Part model, mm, in its own coordinate system. A direction names the side the tool comes from. Round coordinates to 2 decimals unless told otherwise and drop trailing zeros. Loops run counter-clockwise (first coordinate to the right, second up) from the corner with the lowest first, then second, coordinate; pieces in that order, holes last.
from build123d import *
from OCP.BRepFilletAPI import BRepFilletAPI_MakeChamfer

# Parameters (mm, degrees)
SKETCH1_W           = 82
SKETCH1_H           = 30
BOSS_EXTRUDE1_DEPTH = 5
CUT_EXTRUDE1_DEPTH  = 10
CHAMFER1_SIZE       = 0.5
CHAMFER1_SIZE2      = 0.366025404
CUT_EXTRUDE3_REACH  = 89.459
CHAMFER3_SIZE       = 0.5


with BuildPart() as part:
    # Sketch1 → Boss-Extrude1 (new body)
    with BuildSketch(Plane.XY):
        with Locations((41, 15)):
            Rectangle(SKETCH1_W, SKETCH1_H)
    extrude(amount=BOSS_EXTRUDE1_DEPTH)

    # Sketch2 → Cut-Extrude1 (cut)
    with BuildSketch(Plane.XZ):
        Polygon((0.973292227, 5.1), (9.093205081, 5.1), (6.090983681, -0.1), (3.975513627, -0.1), align=None)
        Polygon((9.860043573, -0.1), (17.979956427, -0.1), (14.977735027, 5.1), (12.862264973, 5.1), align=None)
        Polygon((18.743292227, 5.1), (26.863205081, 5.1), (23.860983681, -0.1), (21.745513627, -0.1), align=None)
        Polygon((27.630043573, -0.1), (35.749956427, -0.1), (32.747735027, 5.1), (30.632264973, 5.1), align=None)
        Polygon((36.513292227, 5.1), (44.633205081, 5.1), (41.630983681, -0.1), (39.515513627, -0.1), align=None)
        Polygon((45.400043573, -0.1), (53.519956427, -0.1), (50.517735027, 5.1), (48.402264973, 5.1), align=None)
        Polygon((54.283292227, 5.1), (62.403205081, 5.1), (59.400983681, -0.1), (57.285513627, -0.1), align=None)
        Polygon((63.170043573, -0.1), (71.289956427, -0.1), (68.287735027, 5.1), (66.172264973, 5.1), align=None)
        Polygon((72.053292227, 5.1), (80.173205081, 5.1), (77.170983681, -0.1), (75.055513627, -0.1), align=None)
    extrude(amount=-CUT_EXTRUDE1_DEPTH, mode=Mode.SUBTRACT)

    # Chamfer1: one chamfer whose edges measure the first distance from different faces: ONE call of the kernel's chamfer builder (chamfer() names one face for all edges)
    chamfer1_edges_1 = [part.edges().sort_by_distance(p)[0] for p in [
        (31.69, 10, 5),
        (40.573248654, 10, 5),
        (49.46, 10, 5),
        (58.343248654, 10, 5),
        (8.033248654, 0, 0),
        (67.23, 10, 5),
        (19.805, 0, 0),
        (25.803248654, 0, 0),
        (37.575, 0, 0),
        (76.113248654, 10, 5),
        (43.573248654, 0, 0),
        (55.345, 0, 0),
        (61.343248654, 0, 0),
        (73.115, 0, 0),
        (79.614359354, 0, 0),
        (76.113248654, 10, 0),
        (67.23, 10, 0),
        (58.343248654, 10, 0),
        (49.46, 10, 0),
        (40.573248654, 10, 0),
        (31.69, 10, 0),
        (22.803248654, 10, 0),
        (13.92, 10, 0),
        (5.033248654, 10, 0),
        (10.92, 0, 5),
        (16.918248654, 0, 5),
        (28.69, 0, 5),
        (34.688248654, 0, 5),
        (46.46, 0, 5),
        (52.458248654, 0, 5),
        (64.23, 0, 5),
        (70.228248654, 0, 5),
        (81.057735027, 0, 5),
        (1.9588893, 0, 0),
        (5.033248654, 10, 5),
        (13.92, 10, 5),
        (0.515513627, 0, 5),
        (22.803248654, 10, 5),
    ]]
    chamfer1_edges_2 = [part.edges().sort_by_distance(p)[0] for p in [
        (48.344529946, 5, 5),
    ]]
    chamfer1_side_2 = [part.faces().sort_by_distance(p)[0] for p in [
        (46.901154273, 5, 2.5),
    ]]
    chamfer1_edges_3 = [part.edges().sort_by_distance(p)[0] for p in [
        (50.575470054, 5, 5),
    ]]
    chamfer1_side_3 = [part.faces().sort_by_distance(p)[0] for p in [
        (52.018845727, 5, 2.5),
    ]]
    chamfer1_edges_4 = [part.edges().sort_by_distance(p)[0] for p in [
        (66.114529946, 5, 5),
    ]]
    chamfer1_side_4 = [part.faces().sort_by_distance(p)[0] for p in [
        (64.671154273, 5, 2.5),
    ]]
    chamfer1_edges_5 = [part.edges().sort_by_distance(p)[0] for p in [
        (68.345470054, 5, 5),
    ]]
    chamfer1_side_5 = [part.faces().sort_by_distance(p)[0] for p in [
        (69.788845727, 5, 2.5),
    ]]
    chamfer1_edges_6 = [part.edges().sort_by_distance(p)[0] for p in [
        (77.228718708, 5, 0),
        (74.9977786, 5, 0),
        (59.458718708, 5, 0),
        (57.2277786, 5, 0),
        (41.688718708, 5, 0),
        (39.4577786, 5, 0),
        (23.918718708, 5, 0),
        (21.6877786, 5, 0),
        (6.148718708, 5, 0),
        (3.9177786, 5, 0),
    ]]
    chamfer1_side_6 = [part.faces().sort_by_distance(p)[0] for p in [
        (41.090558892, 17.128531177, 0),
    ]]
    chamfer1_edges_7 = [part.edges().sort_by_distance(p)[0] for p in [
        (12.804529946, 5, 5),
    ]]
    chamfer1_side_7 = [part.faces().sort_by_distance(p)[0] for p in [
        (11.361154273, 5, 2.5),
    ]]
    chamfer1_edges_8 = [part.edges().sort_by_distance(p)[0] for p in [
        (15.035470054, 5, 5),
    ]]
    chamfer1_side_8 = [part.faces().sort_by_distance(p)[0] for p in [
        (16.478845727, 5, 2.5),
    ]]
    chamfer1_edges_9 = [part.edges().sort_by_distance(p)[0] for p in [
        (30.574529946, 5, 5),
    ]]
    chamfer1_side_9 = [part.faces().sort_by_distance(p)[0] for p in [
        (29.131154273, 5, 2.5),
    ]]
    chamfer1_edges_10 = [part.edges().sort_by_distance(p)[0] for p in [
        (32.805470054, 5, 5),
    ]]
    chamfer1_side_10 = [part.faces().sort_by_distance(p)[0] for p in [
        (34.248845727, 5, 2.5),
    ]]
    chamfer1 = BRepFilletAPI_MakeChamfer(part.part.solid().wrapped)
    for e in chamfer1_edges_1:
        chamfer1.Add(CHAMFER1_SIZE, e.wrapped)
    for e in chamfer1_edges_2:
        chamfer1.Add(CHAMFER1_SIZE, CHAMFER1_SIZE2, e.wrapped, chamfer1_side_2[0].wrapped)  # the first distance lies on this face
    for e in chamfer1_edges_3:
        chamfer1.Add(CHAMFER1_SIZE, CHAMFER1_SIZE2, e.wrapped, chamfer1_side_3[0].wrapped)  # the first distance lies on this face
    for e in chamfer1_edges_4:
        chamfer1.Add(CHAMFER1_SIZE, CHAMFER1_SIZE2, e.wrapped, chamfer1_side_4[0].wrapped)  # the first distance lies on this face
    for e in chamfer1_edges_5:
        chamfer1.Add(CHAMFER1_SIZE, CHAMFER1_SIZE2, e.wrapped, chamfer1_side_5[0].wrapped)  # the first distance lies on this face
    for e in chamfer1_edges_6:
        chamfer1.Add(CHAMFER1_SIZE, CHAMFER1_SIZE2, e.wrapped, chamfer1_side_6[0].wrapped)  # the first distance lies on this face
    for e in chamfer1_edges_7:
        chamfer1.Add(CHAMFER1_SIZE, CHAMFER1_SIZE2, e.wrapped, chamfer1_side_7[0].wrapped)  # the first distance lies on this face
    for e in chamfer1_edges_8:
        chamfer1.Add(CHAMFER1_SIZE, CHAMFER1_SIZE2, e.wrapped, chamfer1_side_8[0].wrapped)  # the first distance lies on this face
    for e in chamfer1_edges_9:
        chamfer1.Add(CHAMFER1_SIZE, CHAMFER1_SIZE2, e.wrapped, chamfer1_side_9[0].wrapped)  # the first distance lies on this face
    for e in chamfer1_edges_10:
        chamfer1.Add(CHAMFER1_SIZE, CHAMFER1_SIZE2, e.wrapped, chamfer1_side_10[0].wrapped)  # the first distance lies on this face
    add(Compound.cast(chamfer1.Shape()), mode=Mode.REPLACE)

    # Sketch11 → Cut-Extrude3 (cut, up to next)
    with BuildSketch(Plane.XY.offset(5), mode=Mode.PRIVATE) as cut_extrude3_sk1:
        with BuildLine():
            Line((4, 14), (28, 14))
            ThreePointArc((28, 14), (16, 26), (4, 14))
        make_face()
    cut_extrude3_tool1 = extrude(cut_extrude3_sk1.sketch, amount=-CUT_EXTRUDE3_REACH, mode=Mode.PRIVATE) & part.part
    # Sketch11 → Cut-Extrude3 (cut, up to next)
    with BuildSketch(Plane.XY.offset(5), mode=Mode.PRIVATE) as cut_extrude3_sk2:
        with BuildLine():
            Line((29, 26), (53, 26))
            ThreePointArc((53, 26), (41, 14), (29, 26))
        make_face()
    cut_extrude3_tool2 = extrude(cut_extrude3_sk2.sketch, amount=-CUT_EXTRUDE3_REACH, mode=Mode.PRIVATE) & part.part
    # Sketch11 → Cut-Extrude3 (cut, up to next)
    with BuildSketch(Plane.XY.offset(5), mode=Mode.PRIVATE) as cut_extrude3_sk3:
        with BuildLine():
            Line((54, 14), (78, 14))
            ThreePointArc((78, 14), (66, 26), (54, 14))
        make_face()
    cut_extrude3_tool3 = extrude(cut_extrude3_sk3.sketch, amount=-CUT_EXTRUDE3_REACH, mode=Mode.PRIVATE) & part.part
    add(cut_extrude3_tool1.solids().sort_by_distance((16, 19.092958, 5))[0], mode=Mode.SUBTRACT)
    add(cut_extrude3_tool2.solids().sort_by_distance((41, 20.907042, 5))[0], mode=Mode.SUBTRACT)
    add(cut_extrude3_tool3.solids().sort_by_distance((66, 19.092958, 5))[0], mode=Mode.SUBTRACT)

    # Chamfer3
    chamfer3_edges = [part.edges().sort_by_distance(p)[0] for p in [
        (82, 15.25, 0),
        (0, 15.25, 0),
        (41, 30, 0),
        (0, 15.25, 5),
        (41, 30, 5),
        (41, 14, 5),
        (66, 14, 0),
        (66, 26, 0),
        (66, 14, 5),
        (66, 26, 5),
        (41, 14, 0),
        (41, 26, 0),
        (16, 14, 0),
        (16, 26, 0),
        (16, 14, 5),
        (16, 26, 5),
        (82, 15.25, 5),
    ]]
    chamfer(chamfer3_edges, length=CHAMFER3_SIZE)


solid = part.part
1) Slice it at A-A, the plane x = 41. Give the cut face in (y, z).
Values:
outline: (10, 0.5) - (10.5, 0) - (13.5, 0) - (14, 0.5) - (14, 4.5) - (13.5, 5) - (10.5, 5) - (10, 4.5) - close; (26, 0.5) - (26.5, 0) - (29.5, 0) - (30, 0.5) - (30, 4.5) - (29.5, 5) - (26, 5) - close
2) Slice it at B-B, the plane y = 15. Give the number of separate pieces and of enclosed holes in the cut face, then the cut area to 3 significant figures.
Values:
separate pieces: 4
enclosed holes: 0
area: 120 mm2
3) Mould opens along X. For faces 1 (the face through (34.392, 5.176, 2.252)), 2 (the face through (40, 30, 2)) say: released by +X, released by -X, zero draft, split by the parting line, or undercut.
Values:
face 1: undercut
face 2: zero draft
4) Tool access for faces 3 (the face through (52.162, 5.176, 2.252)), 4 (the face through (16, 26, 3)), 5 (the face through (16.274, 26.132, 0.365)), 6 (the face through (58, 10, 3)): list every direction of +Z, -Z, +X, -X, +Y, -Y with a clear straight run to the whole face (end or side of a thin tool).
Values:
face 3: -Z, -Y
face 4: +Z, -Z
face 5: -Z
face 6: +Z, -Y
5) Wall check: line 1 along Y through (x, z) = (27, 3.5); line 2 along X through (y, z) = (19, 4.2); line 3 along X through (y, z) = (22, 4.05). Give the ranges that are in metal, low to high.
Values:
line 1: y = 0 to 14, 18.8 to 30
line 2: x = 0 to 5.09, 26.91 to 31.25, 50.75 to 55.09, 76.91 to 82
line 3: x = 0 to 7.06, 24.94 to 29.69, 52.31 to 57.06, 74.94 to 82
6) Drop a flat-ended pin along its axis: pin 1 Ø1.2 at (x, z) = (40.5, 3.5) entering from -Y. Give the stop position or say it passes through.
Values:
pin 1: stops at y = 10
